Build history of the part. All positions in model axes, mm. Give positions to 0.01 mm unless a question says otherwise; leave off trailing zeros. Order: outer loops, then holes, each group sorted by start corner. A loop starts at its lowest first (then second) coordinate and runs counter-clockwise, first axis right, second up. Notation, with made-up numbers: M -38,-33.75 L -3,-33.75 A20 ccw -3,-3.75 Z; hole C 8.5,86 d3. An arc over 180 degrees is marked long. One line per item, written item: value. Start each with the question number.
from build123d import *

# Parameters (mm, degrees)
SKETCH2_W           = 32.15
SKETCH2_H           = 15.8
BOSS_EXTRUDE1_DEPTH = 10.4
SKETCH3_R           = 1.7
CUT_EXTRUDE1_DEPTH  = 10.4


with BuildPart() as part:
    # Sketch2 → Boss-Extrude1 (new body)
    with BuildSketch(Plane(origin=(0, 0, 0), x_dir=(1, 0, 0), z_dir=(0, 1, 0))):
        with Locations((16.075, 7.9)):
            Rectangle(SKETCH2_W, SKETCH2_H)
    extrude(amount=BOSS_EXTRUDE1_DEPTH)

    # Sketch3 → Cut-Extrude1 (cut)
    with BuildSketch(Plane(origin=(0, 10.4, 0), x_dir=(1, 0, 0), z_dir=(0, 1, 0))):
        with Locations(Location((3.1, 2.94, 0), (0, 0, 270))):
            Circle(SKETCH3_R)
        with Locations(Location((24.99, 12.78, 0), (0, 0, 270))):
            Circle(SKETCH3_R)
    extrude(amount=-CUT_EXTRUDE1_DEPTH, mode=Mode.SUBTRACT)

    # Sketch13 → Revolve1 (revolve)
    with BuildSketch(Plane(origin=(0, 5.2, 0), x_dir=(1, 0, 0), z_dir=(0, 1, 0))):
        with BuildLine():
            Line((4.870191612, 15.8), (9.470191612, 15.8))
            ThreePointArc((9.470191612, 15.8), (8.487581187, 16.827034892), (7.12986911, 17.247679442))
            Line((7.12986911, 17.247679442), (7.12986911, 17.847679442))
            ThreePointArc((7.12986911, 17.847679442), (6.138456674, 18.695290943), (4.870191612, 19))
            Line((4.870191612, 19), (4.870191612, 15.8))
        make_face()
    revolve(axis=Axis((4.870191612, 5.2, -15.8), (0, 0, -1)))


solid = part.part
1) Slice it at A-A (x = 24.99). List the corners of the cut face in (y, z).
2) Slice it at D-D (y = 7). State how many separate pieces and enclosed holes the cut face has, plus the area to 3 significant figures.
3) Slice it at B-B (z = -12.78). List the corners of the cut face in (x, y).
4) Drop flat-ended pins along their axis: P1, Ø1, axis at x = 28.5, y = 5.5, coming from the -Z side; P2, Ø5, axis at x = 20, z = -17, coming from the +Y side; P3, Ø2.5, axis at x = 24.99, z = -12.78, coming from the +Y side; P4, Ø4, axis at x = 10.5, y = 2.5, coming from the -Z side. Give the stop position or say it passes through.
5) Slice it at C-C (x = 20). List the corners of the cut face in (y, z).
6) Pull direction X, two halves, no side cores. Call faces 1 (the cylindrical face through (4.58, 2.96, -17.55)), 2 (the cylindrical face through (26.676, 5.273, -13.001)), 3 (the flat face through (32.15, 5, -8)): pulls with the +X half, pulls with the -X half, needs draft (parallel to the pull), parting line crosses it, or undercut.
7) Drill centre lines: line 1 (X direction, y = 8.25, z = -3); line 2 (X direction, y = 8, z = -12.78); line 3 (Z direction, x = 18.5, y = 2.75). Where is each one in solid material? Low to high.
Results list:
1. outline: M 0,-15.8 L 10.4,-15.8 L 10.4,-14.48 L 0,-14.48 Z; M 0,-11.08 L 10.4,-11.08 L 10.4,0 L 0,0 Z
2. separate pieces: 1
2. enclosed holes: 2
2. area: 502 mm²
3. outline: M 0,0 L 23.29,0 L 23.29,10.4 L 0,10.4 Z; M 26.69,0 L 32.15,0 L 32.15,10.4 L 26.69,10.4 Z
4. P1: stops at z = -15.8
4. P2: stops at y = 10.4
4. P3: passes through
4. P4: stops at z = -16.3
5. outline: M 0,-15.8 L 10.4,-15.8 L 10.4,0 L 0,0 Z
6. face 1: parting line crosses it
6. face 2: undercut
6. face 3: pulls with the +X half
7. line 1: x = 0 to 1.4, 4.8 to 32.15
7. line 2: x = 0 to 23.29, 26.69 to 32.15
7. line 3: z = -15.8 to 0
